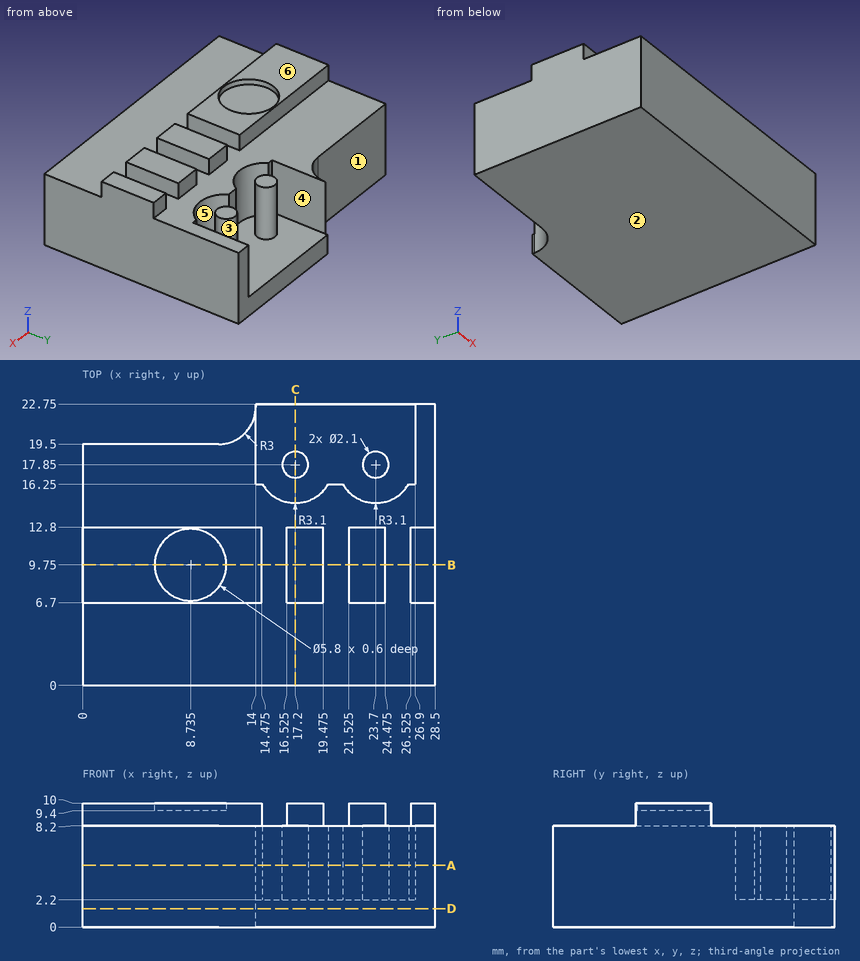
Check sheet for the drawn part. Datum: minimum x, y, z corner. Units: mm. A direction names the side the tool comes from. Round coordinates to 2 decimals unless told otherwise and drop trailing zeros. Write each loop counter-clockwise with the first axis right and the second up, starting at its lowest first coordinate (ties: lowest second). Pieces come first, ordered by that corner, then holes. Notation, with made-up numbers: (35.25, 49.5) -> (82.25, 49.5) arc R35 ccw to (82.25, 81.5) -> close; hole circle Ø10 at (26.25, 4). An arc over 180 degrees is marked (long way). One line per item, written item: value. Start each with the question number.
(1) Cross-section at C-C, the plane x = 17.2. Record the cut outline in (y, z).
(2) Go/stop test with flat-tipped pins: pin 1 Ø4 at (x, z) = (25.5, 8) entering from -Y; pin 2 Ø1.1 at (x, y) = (24, 17.5) entering from +Z; pin 3 Ø2.5 at (x, y) = (19, 20) entering from +Z; pin 4 Ø0.9 at (x, z) = (18, 9) entering from -Y. Record where each tip stops, or that it passes through.
(3) Cross-section at A-A, the plane z = 5. Record the cut outline in (x, y), and give its area (3 significant figures).
(4) Cross-section at B-B, the plane y = 9.75. Record the cut outline in (x, z) (3 decimals), and give its area (3 significant figures).
(5) Cross-section at D-D, the plane z = 1.5. Record the cut outline in (x, y).
(6) Access from +Z, -Z, +X, -X, +Y, -Y to the whole of each face (thin tool, end or side, straight path). Record for the marked faces 4, 5 and 6.
(7) Draft check along Y on the marked faces 1, 2 and 3. Enter one of: +Y half, -Y half, draft (parallel to the pull), parting line (faces both ways), or undercut.
(8) Scan lines: line 1 (X direction, y = 9, z = 8.5) (3 decimals); line 2 (Y direction, x = 17.5, z = 9); line 3 (Y direction, x = 16.75, z = 7). Record each from-to range of solid material in increasing order. Write a range as [from, to].
Answer:
1. outline: (0, 0) -> (22.75, 0) -> (22.75, 2.2) -> (18.9, 2.2) -> (18.9, 8.2) -> (16.8, 8.2) -> (16.8, 2.2) -> (14.75, 2.2) -> (14.75, 8.2) -> (12.8, 8.2) -> (12.8, 10) -> (6.7, 10) -> (6.7, 8.2) -> (0, 8.2) -> close
2. pin 1: y = 0
2. pin 2: z = 8.2
2. pin 3: z = 2.2
2. pin 4: y = 6.7
3. outline: (0, 0) -> (28.5, 0) -> (28.5, 22.75) -> (26.9, 22.75) -> (26.9, 16.25) -> (26.36, 16.25) arc R3.1 cw to (21.04, 16.25) -> (19.86, 16.25) arc R3.1 cw to (14.54, 16.25) -> (14, 16.25) -> (14, 22.5) arc R3 cw to (11, 19.5) -> (0, 19.5) -> close; circle Ø2.1 at (17.2, 17.85); circle Ø2.1 at (23.7, 17.85)
3. area: 517 mm²
4. outline: (0, 0) -> (28.5, 0) -> (28.5, 10) -> (26.525, 10) -> (26.525, 8.2) -> (24.475, 8.2) -> (24.475, 10) -> (21.525, 10) -> (21.525, 8.2) -> (19.475, 8.2) -> (19.475, 10) -> (16.525, 10) -> (16.525, 8.2) -> (14.475, 8.2) -> (14.475, 10) -> (11.635, 10) -> (11.635, 9.4) -> (5.835, 9.4) -> (5.835, 10) -> (0, 10) -> close
4. area: 270 mm²
5. outline: (0, 0) -> (28.5, 0) -> (28.5, 22.75) -> (14, 22.75) -> (14, 22.5) arc R3 cw to (11, 19.5) -> (0, 19.5) -> close
6. face 4: +Z, +Y
6. face 5: +Z
6. face 6: +Z, +X, -X, +Y, -Y
7. face 1: +Y half
7. face 2: draft
7. face 3: undercut
8. line 1: [0, 14.475], [16.525, 19.475], [21.525, 24.475], [26.525, 28.5]
8. line 2: [6.7, 12.8]
8. line 3: [0, 14.78], [16.9, 18.8]
